from build123d import *

# Parameters (mm, degrees)
F1_DEPTH = 90
F2_R     = 5
F4_DEPTH = 10
F6_DEPTH = 60.001


with BuildPart() as f1:
    # F0 (on Top) → F1 (new body)
    with BuildSketch(Plane.XY):
        Polygon((17.489978, -16.504586), (17.489978, -21.504586), (37.489978, -21.504586), (37.489978, -13.504586), (-22.510022, -13.504586), (-22.510022, -21.504586), (-2.510022, -21.504586), (-2.510022, -16.504586), align=None)
    extrude(amount=F1_DEPTH)

    # F2
    f2_edges = [f1.edges().sort_by_distance(p)[0] for p in [
        (-22.510022, -17.504586, 0),
        (37.489978, -17.504586, 0),
    ]]
    fillet(f2_edges, radius=F2_R)

    # F3 (on face) → F4 (join)
    with BuildSketch(Plane(origin=(0, -13.504586, 0), x_dir=(-1, 0, 0), z_dir=(0, 1, 0))):
        with BuildLine():
            Line((22.510022, 5), (22.510022, 20))
            Line((22.510022, 20), (-37.489978, 20))
            Line((-37.489978, 20), (-37.489978, 5))
            ThreePointArc((-37.489978, 5), (-36.025512, 1.464466), (-32.489978, 0))
            Line((-32.489978, 0), (17.510022, 0))
            ThreePointArc((17.510022, 0), (21.045556, 1.464466), (22.510022, 5))
        make_face()
    extrude(amount=F4_DEPTH)

    # F5 (on face) → F6 (cut, through all)
    with BuildSketch(Plane.YZ.offset(37.489978)):
        Polygon((-13.504586, 10), (-3.504586, 14.040262), (-3.504586, 20), (-13.504586, 20), align=None)
    extrude(amount=-F6_DEPTH, mode=Mode.SUBTRACT)


solid = f1.part
Read the model definition and answer for the solid it produces. Units are mm, in the model's axes. A direction names the side the tool comes from. Give positions to 0.01 mm unless a question says otherwise; leave off trailing zeros. Loops run counter-clockwise (first coordinate to the right, second up) from the corner with the lowest first, then second, coordinate; pieces in that order, holes last. Notation, with made-up numbers: (-35.5, 28.25) -> (12.5, 28.25) arc R23 ccw to (12.5, 57.25) -> close; hole circle Ø8 at (-39.5, 1). An arc over 180 degrees is marked (long way). Answer as CSV lines item,"result".
Item 1: For faces 1 (the face through (7, -16.505, 44)), 2 (the face through (7.91, -8.575, 11.992)), 3 (the face through (8, -13, 0)), determine the directions among +Z, -Z, +X, -X, +Y, -Y from which every point of the face is accessible in a straight line to the end or side of a thin tool.
Returned:
face 1,"+Z, -Z, -Y"
face 2,"+Z, +X, -X"
face 3,"-Z, +X, -X, +Y, -Y"
Item 2: Determine the mould class of faces 4 (the face through (7, -16, 90)), 5 (the face through (-22.51, -17, 47)), 6 (the face through (17.49, -19, 44)) for opening direction X: +X half, -X half, draft (parallel to the pull), parting line (faces both ways), or undercut.
Returned:
face 4,"draft"
face 5,"-X half"
face 6,"undercut"
Item 3: Find section C-C on y = -7. Give the vertices of the cut face in (x, z).
Returned:
outline,"(-22.51, 5) arc R5 ccw to (-17.51, 0) -> (32.49, 0) arc R5 ccw to (37.49, 5) -> (37.49, 12.63) -> (-22.51, 12.63) -> close"
Item 4: Each of these flat-tipped pins is pushed along its axis until it touches: pin 1 (10 mm diameter, centred on x = 9, z = 55, fed in from -Y); pin 2 (2 mm diameter, centred on x = -6.5, y = -7.5, fed in from +Z). Where does it stop, or does it pass through?
Returned:
pin 1,"stops at y = -16.5"
pin 2,"stops at z = 12.83"
Item 5: Find section B-B on x = 5. Give the vertices of the cut face in (y, z).
Returned:
outline,"(-16.5, 0) -> (-3.5, 0) -> (-3.5, 14.04) -> (-13.5, 10) -> (-13.5, 90) -> (-16.5, 90) -> close"
Item 6: Find section A-A on z = 80. Give the vertices of the cut face in (x, y), plus the area to 3 significant figures.
Returned:
outline,"(-22.51, -21.5) -> (-2.51, -21.5) -> (-2.51, -16.5) -> (17.49, -16.5) -> (17.49, -21.5) -> (37.49, -21.5) -> (37.49, -13.5) -> (-22.51, -13.5) -> close"
area,"380 mm²"
Item 7: Consider line 1 (X direction, y = -17.5, z = 48.5); line 2 (Y direction, x = -7, z = 28.5); line 3 (Y direction, x = 12.5, z = 62). Determine where each line is inside the solid, lowest interval first. Write a range as [from, to].
Returned:
line 1,"x = [-22.51, -2.51], [17.49, 37.49]"
line 2,"y = [-21.5, -13.5]"
line 3,"y = [-16.5, -13.5]"
